Build history of the part. All positions in model axes, mm. Give positions to 0.01 mm unless a question says otherwise; leave off trailing zeros. Order: outer loops, then holes, each group sorted by start corner. A loop starts at its lowest first (then second) coordinate and runs counter-clockwise, first axis right, second up. Notation, with made-up numbers: (-35, -5) - (9, -5) arc R18 ccw to (9, 29) - close; hole circle Ø6 at (-35, -40). An arc over 180 degrees is marked (long way). Use a Markdown table: item, result.
from build123d import *

# Parameters (mm, degrees)
F0_W     = 410.845
F0_H     = 673.883108
F1_DEPTH = 50.8
F2_R     = 20.097435
F3_DEPTH = 33.782
F4_R     = 17.468499
F5_DEPTH = 38.1


with BuildPart() as f1:
    # F0 (on Front) → F1 (new body)
    with BuildSketch(Plane.XZ):
        Rectangle(F0_W, F0_H)
    extrude(amount=F1_DEPTH)

    # F2 (on face) → F3 (join)
    with BuildSketch(Plane(origin=(0, 0, -336.941554), x_dir=(1, 0, 0), z_dir=(0, 0, -1))):
        with Locations((-176.623374, 26.477363)):
            Circle(F2_R)
    extrude(amount=F3_DEPTH)

    # F4 (on face) → F5 (join)
    with BuildSketch(Plane.XY.offset(336.941554)):
        with Locations((173.230782, -25.4)):
            Circle(F4_R)
    extrude(amount=F5_DEPTH)


solid = f1.part
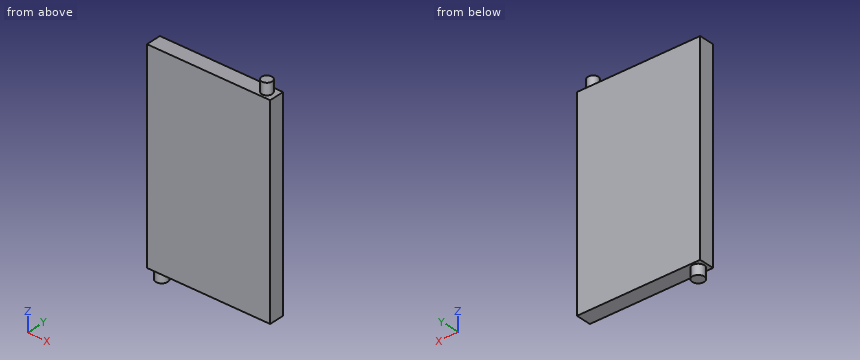
1) Slice it at C-C (x = 174.5). Write the cut outline in (y, z).
Computed:
| item | result |
|---|---|
| outline | (-50.8, -336.94) - (0, -336.94) - (0, 336.94) - (-7.98, 336.94) - (-7.98, 375.04) - (-42.82, 375.04) - (-42.82, 336.94) - (-50.8, 336.94) - close |
2) Slice it at A-A (y = -36). Write the cut outline in (x, z).
Computed:
| item | result |
|---|---|
| outline | (-205.42, -336.94) - (-194.32, -336.94) - (-194.32, -370.72) - (-158.93, -370.72) - (-158.93, -336.94) - (205.42, -336.94) - (205.42, 336.94) - (187.12, 336.94) - (187.12, 375.04) - (159.35, 375.04) - (159.35, 336.94) - (-205.42, 336.94) - close |
3) Wall check: line 1 (Z direction, x = 93, y = -42); line 2 (Z direction, x = -188, y = -22). Give the ranges that are in metal, low to high. Write a range as from..to.
Computed:
| item | result |
|---|---|
| line 1 | z = -336.94..336.94 |
| line 2 | z = -370.72..336.94 |
4) Pin check, flat tips, straight feed: P1, Ø8, axis at x = -94.5, y = -31, coming from the +Z side; P2, Ø1, axis at x = 45.5, y = -43, coming from the -Z side. Stop position of each tip, or through.
Computed:
| item | result |
|---|---|
| P1 | stops at z = 336.94 |
| P2 | stops at z = -336.94 |
5) Slice it at B-B (x = -95.5). Write the cut outline in (y, z).
Computed:
| item | result |
|---|---|
| outline | (-50.8, -336.94) - (0, -336.94) - (0, 336.94) - (-50.8, 336.94) - close |
